```python
from build123d import *

# Parameters (mm, degrees)
SKETCH1_W                              = 165
SKETCH1_H                              = 165
BOSS_EXTRUDE1_DEPTH                    = 38
SKETCH2_W                              = 95
SKETCH2_H                              = 95
BOSS_EXTRUDE2_DEPTH                    = 38
BOSS_EXTRUDE4_DEPTH                    = 95
SKETCH5_R                              = 12.7
CUT_EXTRUDE1_DEPTH                     = 198.379076905
CUT_EXTRUDE2_DEPTH                     = 222.998873871
CUT_EXTRUDE2_DEPTH_BACK                = 222.998873871
FILLET1_R                              = 10
FILLET2_R                              = 10
SKETCH9_R                              = 26
CUT_EXTRUDE3_DEPTH                     = 36.83
SKETCH10_R                             = 76.2
SKETCH10_R_2                           = 69.85
CUT_EXTRUDE4_DEPTH                     = 10
F_1_2_14_NPSM_TAPPED_HOLE1_D           = 18.9738
F_1_2_14_NPSM_TAPPED_HOLE1_DEPTH       = 63.5
F_1_2_14_NPSM_TAPPED_HOLE1_CSINK_D     = 22.1742
F_1_2_14_NPSM_TAPPED_HOLE1_CSINK_ANGLE = 90
F_1_2_14_NPSM_TAPPED_HOLE1_TIP         = 5.700304607
SKETCH13_R                             = 6.35
CUT_EXTRUDE5_DEPTH                     = 25
SKETCH14_R                             = 6.35
CUT_EXTRUDE7_DEPTH                     = 170.896291896


with BuildPart() as part:
    # Sketch1 → Boss-Extrude1 (new body)
    with BuildSketch(Plane(origin=(0, 0, 0), x_dir=(1, 0, 0), z_dir=(0, 1, 0))):
        Rectangle(SKETCH1_W, SKETCH1_H)
    extrude(amount=BOSS_EXTRUDE1_DEPTH)

    # Sketch2 → Boss-Extrude2 (add)
    with BuildSketch(Plane(origin=(0, 38, 0), x_dir=(1, 0, 0), z_dir=(0, 1, 0))):
        Rectangle(SKETCH2_W, SKETCH2_H)
    extrude(amount=BOSS_EXTRUDE2_DEPTH)

    # Sketch3 → Boss-Extrude4 (add)
    with BuildSketch(Plane(origin=(0, 0, -47.5), x_dir=(-1, 0, 0), z_dir=(0, 0, -1))):
        with BuildLine():
            Line((-47.5, 76), (47.5, 76))
            ThreePointArc((47.5, 76), (0, 123.5), (-47.5, 76))
        make_face()
    extrude(amount=-BOSS_EXTRUDE4_DEPTH)

    # Sketch5 → Cut-Extrude1 (cut, through all)
    with BuildSketch(Plane(origin=(0, 0, -47.5), x_dir=(-1, 0, 0), z_dir=(0, 0, -1))):
        with Locations((0, 76)):
            Circle(SKETCH5_R)
    extrude(amount=-CUT_EXTRUDE1_DEPTH, mode=Mode.SUBTRACT)

    # Sketch8 → Cut-Extrude2 (cut, two sides: drawn at the far end of the back side and taken through both)
    with BuildSketch(Plane(origin=(82.5, 0, 0), x_dir=(0, 0, -1), z_dir=(1, 0, 0)).offset(-CUT_EXTRUDE2_DEPTH_BACK)):
        Polygon((-19.102036328, 453.345111178), (-19.102036328, 123.5), (-19.102036328, 100.748776974), (-19.102036328, 38), (19.102036328, 38), (19.102036328, 100.748776974), (19.102036328, 123.5), (19, 123.5), (-19, 123.5), (-348.845111178, 123.5), (117.698474691, -342.899262388), (447.44154954, -13.05415121), align=None)
    extrude(amount=CUT_EXTRUDE2_DEPTH + CUT_EXTRUDE2_DEPTH_BACK, mode=Mode.SUBTRACT)

    # Fillet1
    fillet1_edges = [part.edges().sort_by_distance(p)[0] for p in [
        (82.5, 19, 82.5),
    ]]
    fillet(fillet1_edges, radius=FILLET1_R)

    # Fillet2
    fillet2_edges = [part.edges().sort_by_distance(p)[0] for p in [
        (-82.5, 19, 82.5),
        (-82.5, 19, -82.5),
        (82.5, 19, -82.5),
    ]]
    fillet(fillet2_edges, radius=FILLET2_R)

    # Sketch9 → Cut-Extrude3 (cut)
    with BuildSketch(Plane.XZ):
        with Locations(Location((0, 0, 0), (0, 0, 270))):
            Circle(SKETCH9_R)
    extrude(amount=-CUT_EXTRUDE3_DEPTH, mode=Mode.SUBTRACT)

    # Sketch10 → Cut-Extrude4 (cut)
    with BuildSketch(Plane.XZ):
        with Locations(Location((0, 0, 0), (0, 0, 270))):
            Circle(SKETCH10_R)
        with Locations(Location((0, 0, 0), (0, 0, 270))):
            Circle(SKETCH10_R_2, mode=Mode.SUBTRACT)
    extrude(amount=-CUT_EXTRUDE4_DEPTH, mode=Mode.SUBTRACT)

    # 1/2-14 NPSM Tapped Hole1
    with Locations(Plane(origin=(-0.938861221, 19, -82.5), x_dir=(-1, 0, 0), z_dir=(0, 0, -1))):
        with Locations((0, 0)):
            CounterSinkHole(F_1_2_14_NPSM_TAPPED_HOLE1_D / 2, F_1_2_14_NPSM_TAPPED_HOLE1_CSINK_D / 2, depth=F_1_2_14_NPSM_TAPPED_HOLE1_DEPTH, counter_sink_angle=F_1_2_14_NPSM_TAPPED_HOLE1_CSINK_ANGLE)
            with Locations((0, 0, -(F_1_2_14_NPSM_TAPPED_HOLE1_DEPTH + F_1_2_14_NPSM_TAPPED_HOLE1_TIP / 2))):  # 118° drill point
                Cone(0, F_1_2_14_NPSM_TAPPED_HOLE1_D / 2, F_1_2_14_NPSM_TAPPED_HOLE1_TIP, mode=Mode.SUBTRACT)

    # Sketch13 → Cut-Extrude5 (cut)
    with BuildSketch(Plane.XZ):
        with Locations(Location((0, -50.5, 0), (0, 0, 270))):
            Circle(SKETCH13_R)
    extrude(amount=-CUT_EXTRUDE5_DEPTH, mode=Mode.SUBTRACT)

    # Sketch14 → Cut-Extrude7 (cut, through all)
    with BuildSketch(Plane.XZ):
        with Locations(Location((-69.30177445, 53.630970139, 0), (0, 0, 270))):
            Circle(SKETCH14_R)
        with Locations(Location((-69.30177445, -53.630970139, 0), (0, 0, 270))):
            Circle(SKETCH14_R)
        with Locations(Location((69.30177445, -53.630970139, 0), (0, 0, 270))):
            Circle(SKETCH14_R)
        with Locations(Location((69.30177445, 53.630970139, 0), (0, 0, 270))):
            Circle(SKETCH14_R)
    extrude(amount=-CUT_EXTRUDE7_DEPTH, mode=Mode.SUBTRACT)


solid = part.part
```
CAD build for the part. Positions are in the model's coordinates, mm. A direction names the side the tool comes from. Coordinates: 2 decimals unless noted, no trailing zeros. Order: outer loops, then holes, each group sorted by start corner. A loop starts at its lowest first (then second) coordinate and runs counter-clockwise, first axis right, second up. Notation, with made-up numbers: M 35.5,10 L 93.5,10 A25 cw 93.5,25 Z; hole C -26,51.25 d3. An arc over 180 degrees is marked long. Answer as CSV lines item,"result".
1) 3-axis set-ups, long thin cutter, end or side, ignore diameter. For faces 1 (the flat face through (47.5, 57, 33)), 2 (the flat face through (-47.5, 57, 33)), 3 (the cylindrical face through (-46.367, 4.93, 60.47)), 4 (the cylindrical face through (-2.174, 28.406, -51.959)), 5 (the flat face through (-1, 91, 19.102)): which of +Z, -Z, +X, -X, +Y, -Y reach the whole face in a straight line?
Verdict:
face 1,"+Z, -Z, +X, +Y"
face 2,"+Z, -Z, -X, +Y"
face 3,"-Y"
face 4,"-Z"
face 5,"+X, -X, +Y"
2) Cut at D-D (y = 19). List the corners of the cut face in (x, z).
Verdict:
outline,"M -82.5,-72.5 A10 ccw -72.5,-82.5 L -12.03,-82.5 L -10.43,-80.9 L -10.43,-23.82 A26 cw long 8.55,-24.55 L 8.55,-80.9 L 10.15,-82.5 L 72.5,-82.5 A10 ccw 82.5,-72.5 L 82.5,72.5 A10 ccw 72.5,82.5 L -72.5,82.5 A10 ccw -82.5,72.5 Z; hole C -69.3,-53.63 d12.7; hole C -69.3,53.63 d12.7; hole C 69.3,-53.63 d12.7; hole C 69.3,53.63 d12.7"
3) Mould opens along Y. For faces 6 (the flat face through (-17, 10, 68)), 7 (the cylindrical face through (1.653, 88.592, 33.102)), 8 (the flat face through (47.5, 57, -33)), 9 (the cylindrical face through (-1.04, 123.49, 33.1)) say: released by +Y, released by -Y, zero draft, split by the parting line, or undercut.
Verdict:
face 6,"released by -Y"
face 7,"undercut"
face 8,"zero draft"
face 9,"released by +Y"
4) Drill centre lines: L1, parallel to Z at x = -12.5, y = 97; L2, parallel to Y at x = 20.5, z = 0; L3, parallel to X at y = 8.5, z = 5. Where is each one in solid material? Low to high. Write a range as from..to.
Verdict:
L1,"-47.5..-19.1, 19.1..47.5"
L2,"36.83..38"
L3,"-82.5..-76.04, -69.67..-25.51, 25.51..69.67, 76.04..82.5"
5) Cut at A-A (y = 55). List the corners of the cut face in (x, z).
Verdict:
outline,"M -47.5,-47.5 L 47.5,-47.5 L 47.5,-19.1 L -47.5,-19.1 Z; M -47.5,19.1 L 47.5,19.1 L 47.5,47.5 L -47.5,47.5 Z"
6) Cut at B-B (z = 0). List the corners of the cut face in (x, y).
Verdict:
outline,"M -82.5,0 L -76.2,0 L -76.2,10 L -69.85,10 L -69.85,0 L -26,0 L -26,36.83 L 26,36.83 L 26,0 L 69.85,0 L 69.85,10 L 76.2,10 L 76.2,0 L 82.5,0 L 82.5,38 L -82.5,38 Z"
7) Cut at C-C (z = -29). List the corners of the cut face in (x, y), then the cut area to 3 significant figures.
Verdict:
outline,"M -82.5,0 L -70.47,0 L -70.47,10 L -63.55,10 L -63.55,0 L 63.55,0 L 63.55,10 L 70.47,10 L 70.47,0 L 82.5,0 L 82.5,38 L 47.5,38 L 47.5,76 A47.5 ccw -47.5,76 L -47.5,38 L -82.5,38 Z; hole C 0,76 d25.4; hole C -0.94,19 d18.97"
area,"12,500 mm2"
8) Flat gauge pins, fed straight in: P1, Ø8, axis at x = 35, y = 99.5, coming from the -Z side; P2, Ø2, axis at x = 25, y = 41.5, coming from the +Z side; P3, Ø4, axis at x = -51.5, z = -53, coming from the +Y side. Where does each tip first touch, or does it go through?
Verdict:
P1,"z = -47.5"
P2,"z = 47.5"
P3,"y = 38"
